Input: part model. Units: mm. Frame: model coordinates. Give positions to 0.01 mm unless a question says otherwise; leave off trailing zeros. Loops run counter-clockwise (first coordinate to the right, second up) from the corner with the lowest first, then second, coordinate; pieces in that order, holes last. Notation, with made-up numbers: M -31,84.5 L -26,84.5 A34 ccw -26,122.5 Z; hole C 1.5,60 d11. An arc over 180 degrees is marked long. Answer as a JSON object with one key per item and string values. Group by question number.
```python
from build123d import *

# Parameters (mm, degrees)
SKETCH1_W                                  = 406.4
SKETCH1_H                                  = 152.4
SKETCH1_W_2                                = 381
SKETCH1_H_2                                = 127
BOSS_EXTRUDE1_DEPTH                        = 12.7
SKETCH2_W                                  = 12.7
SKETCH2_H                                  = 12.7
BOSS_EXTRUDE2_DEPTH                        = 146.05
MIRROR1_AT_THE_SECOND_PLANE_COPY_1_SKETC_W = 12.7
MIRROR1_AT_THE_SECOND_PLANE_COPY_1_SKETC_H = 12.7
MIRROR1_AT_THE_SECOND_PLANE_COPY_1_DEPTH   = 146.05
SKETCH3_W                                  = 406.4
SKETCH3_H                                  = 152.4
SKETCH3_W_2                                = 381
SKETCH3_H_2                                = 127
BOSS_EXTRUDE3_DEPTH                        = 6.35
SKETCH4_W                                  = 406.4
SKETCH4_H                                  = 158.75
BOSS_EXTRUDE4_DEPTH                        = 12.7
SKETCH6_W                                  = 12.7
SKETCH6_H                                  = 12.7
CUT_EXTRUDE1_DEPTH                         = 127
BOSS_EXTRUDE6_DEPTH                        = 127


with BuildPart() as part:
    # Sketch1 → Boss-Extrude1 (new body)
    with BuildSketch(Plane(origin=(0, 0, 0), x_dir=(1, 0, 0), z_dir=(0, 1, 0))):
        Rectangle(SKETCH1_W, SKETCH1_H)
        Rectangle(SKETCH1_W_2, SKETCH1_H_2, mode=Mode.SUBTRACT)
    extrude(amount=BOSS_EXTRUDE1_DEPTH)

    # Sketch2 → Boss-Extrude2 (add)
    with BuildSketch(Plane(origin=(0, 12.7, 0), x_dir=(1, 0, 0), z_dir=(0, 1, 0))):
        with Locations((-196.85, -69.85)):
            Rectangle(SKETCH2_W, SKETCH2_H)
    boss_extrude2 = extrude(amount=BOSS_EXTRUDE2_DEPTH)

    # Mirror1: Boss-Extrude2 across plane
    add(boss_extrude2.mirror(Plane(origin=(0, 0, 0), x_dir=(0, 0, 1), z_dir=(1, 0, 0))))

    # Mirror1 at the second plane: Boss-Extrude2 across plane
    add(boss_extrude2.mirror(Plane.XY))

    # Mirror1 at the second plane copy 1 sketc → Mirror1 at the second plane copy 1 (add)
    with BuildSketch(Plane(origin=(0, 12.7, 0), x_dir=(-1, 0, 0), z_dir=(0, 1, 0))):
        with Locations((-196.85, -69.85)):
            Rectangle(MIRROR1_AT_THE_SECOND_PLANE_COPY_1_SKETC_W, MIRROR1_AT_THE_SECOND_PLANE_COPY_1_SKETC_H)
    extrude(amount=MIRROR1_AT_THE_SECOND_PLANE_COPY_1_DEPTH)

    # Sketch3 → Boss-Extrude3 (add)
    with BuildSketch(Plane(origin=(0, 158.75, 0), x_dir=(1, 0, 0), z_dir=(0, 1, 0))):
        Rectangle(SKETCH3_W, SKETCH3_H)
        Rectangle(SKETCH3_W_2, SKETCH3_H_2, mode=Mode.SUBTRACT)
    extrude(amount=-BOSS_EXTRUDE3_DEPTH)

    # Sketch4 → Boss-Extrude4 (add)
    with BuildSketch(Plane(origin=(0, 0, -76.2), x_dir=(-1, 0, 0), z_dir=(0, 0, -1))):
        with Locations((0, 79.375)):
            Rectangle(SKETCH4_W, SKETCH4_H)
    extrude(amount=-BOSS_EXTRUDE4_DEPTH)

    # Sketch6 → Cut-Extrude1 (cut)
    with BuildSketch(Plane.XY.offset(-63.5)):
        with Locations((-196.85, 6.35)):
            Rectangle(SKETCH6_W, SKETCH6_H)
    extrude(amount=CUT_EXTRUDE1_DEPTH, mode=Mode.SUBTRACT)

    # Sketch5 → Boss-Extrude6 (add)
    with BuildSketch(Plane.XY.offset(-63.5)):
        Polygon((190.5, 12.7), (-190.5, 0), (190.5, 0), align=None)
    extrude(amount=BOSS_EXTRUDE6_DEPTH)


solid = part.part
```
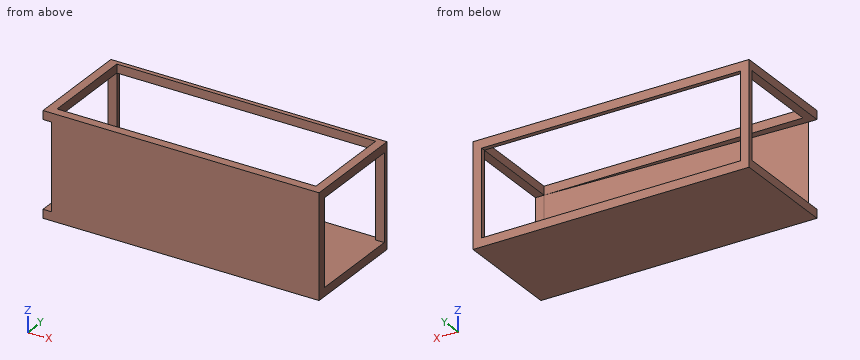
1. Material intervals for L1, parallel to X at y = 48.5, z = 67; L2, parallel to Z at x = 3, y = 27; L3, parallel to Z at x = -151.5, y = 7, sorted ascending.
2. Section A-A (y = 60.5). Output: boundary loops of the cut face in (x, z).
3. Section D-D (x = 102). Output: boundary loops of the cut face in (y, z), then the cut area to 3 significant figures.
4. Section B-B (z = 26). Output: boundary loops of the cut face in (x, y).
5. Section C-C (x = 159). Output: boundary loops of the cut face in (y, z).
6. First-contact query: P1, Ø6, axis at x = 127.5, z = 25, coming from the +Y side; P2, Ø8, axis at y = 77, z = 56.5, coming from the +X side; P3, Ø5, axis at x = 57.5, y = 104, coming from the +Z side; P4, Ø6.5, axis at x = -195.5, z = -31, coming from the -Y side. Flat tips, straight axial feed; report the tip coordinate or a pass-through.
Geometry results:
{
 "1": {"L1": "-203.2 to -190.5, 190.5 to 203.2", "L2": "-76.2 to -63.5", "L3": "-76.2 to -63.5, 63.5 to 76.2"},
 "2": {"outline": "M -203.2,-76.2 L 203.2,-76.2 L 203.2,-63.5 L -203.2,-63.5 Z; M -203.2,63.5 L -190.5,63.5 L -190.5,76.2 L -203.2,76.2 Z; M 190.5,63.5 L 203.2,63.5 L 203.2,76.2 L 190.5,76.2 Z"},
 "3": {"outline": "M 0,-76.2 L 158.75,-76.2 L 158.75,-63.5 L 9.75,-63.5 L 9.75,63.5 L 12.7,63.5 L 12.7,76.2 L 0,76.2 Z; M 152.4,63.5 L 158.75,63.5 L 158.75,76.2 L 152.4,76.2 Z", "area": "3,500 mm2"},
 "4": {"outline": "M -203.2,152.4 L -190.5,152.4 L -190.5,158.75 L -203.2,158.75 Z; M -190.5,0 L 203.2,0 L 203.2,12.7 L 190.5,12.7 Z; M 190.5,152.4 L 203.2,152.4 L 203.2,158.75 L 190.5,158.75 Z"},
 "5": {"outline": "M 0,-76.2 L 158.75,-76.2 L 158.75,-63.5 L 11.65,-63.5 L 11.65,63.5 L 12.7,63.5 L 12.7,76.2 L 0,76.2 Z; M 152.4,63.5 L 158.75,63.5 L 158.75,76.2 L 152.4,76.2 Z"},
 "6": {"P1": "y = 10.7", "P2": "through", "P3": "z = -63.5", "P4": "y = 152.4"}
}
